The listing builds one solid part. Answer for the finished solid, in the listing's coordinates (mm). Face numbers are marked on the shaded views. A direction names the side the tool comes from. Coordinates: 2 decimals unless noted, no trailing zeros. Order: outer loops, then holes, each group sorted by start corner. A loop starts at its lowest first (then second) coordinate and runs counter-clockwise, first axis right, second up. Notation, with made-up numbers: (42.25, 60) -> (77.25, 60) arc R11 cw to (77.25, 79) -> close; hole circle Ø7 at (55.5, 38.25). An arc over 180 degrees is marked (long way). Return JSON: item names as keys, results as strings.
from build123d import *

# Parameters (mm, degrees)
F0_R     = 19.05
F2_DEPTH = 6.35
F1_R     = 3.175
F3_DEPTH = 19.05
F4_R     = 3.302
F5_DEPTH = 25.4


with BuildPart() as f2:
    # F0 (on Front) → F2 (new body)
    with BuildSketch(Plane.XZ):
        Circle(F0_R)
    extrude(amount=F2_DEPTH)

    # F1 (on Front) → F3 (join)
    with BuildSketch(Plane.XZ):
        with Locations((4.173186, 11.943939)):
            Circle(F1_R)
        with Locations((-11.943939, 4.173186)):
            Circle(F1_R)
        with Locations((-4.173186, -11.943939)):
            Circle(F1_R)
        with Locations((11.943939, -4.173186)):
            Circle(F1_R)
    extrude(amount=F3_DEPTH)

    # F4 (on face) → F5 (cut)
    with BuildSketch(Plane.XZ.offset(6.35)):
        Circle(F4_R)
    extrude(amount=-F5_DEPTH, mode=Mode.SUBTRACT)


solid = f2.part
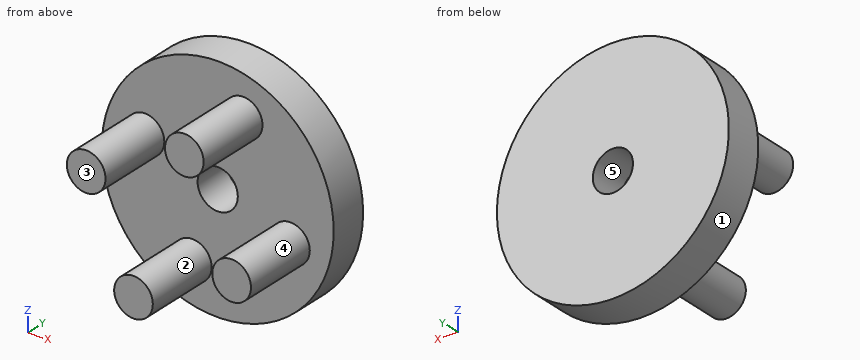
1. The part is cut by section D-D on x = 6.5. Give the vertices of the cut face in (y, z).
Answer block:
{"outline": "(-19.05, 9.78) -> (-6.35, 9.78) -> (-6.35, -17.91) -> (0, -17.91) -> (0, 17.91) -> (-6.35, 17.91) -> (-6.35, 14.1) -> (-19.05, 14.1) -> close"}
2. The part is cut by section B-B on z = 0. Give the vertices of the cut face in (x, y), and give its area (3 significant figures).
Answer block:
{"outline": "(-19.05, -6.35) -> (-3.3, -6.35) -> (-3.3, 0) -> (-19.05, 0) -> close; (3.3, -6.35) -> (19.05, -6.35) -> (19.05, 0) -> (3.3, 0) -> close", "area": "200 mm2"}
3. For the marked faces 1 and 2, determine the directions among +Z, -Z, +X, -X, +Y, -Y from which every point of the face is accessible in a straight line to the end or side of a thin tool.
Answer block:
{"face 1": "+Y, -Y", "face 2": "-Y"}
4. Consider line 1 (Z direction, x = 0, y = -2); line 2 (Y direction, x = 2.5, z = -13); line 3 (X direction, y = -10.75, z = 4). Determine where each line is inside the solid, lowest interval first. Write a range as from..to.
Answer block:
{"line 1": "z = -19.05..-3.3, 3.3..19.05", "line 2": "y = -6.35..0", "line 3": "x = -15.11..-8.77"}
5. The part is cut by section C-C on y = -3.5. Give the vertices of the cut face in (x, z), and give its area (3 significant figures).
Answer block:
{"outline": "circle Ø38.1 at (0, 0); hole circle Ø6.6 at (0, 0)", "area": "1,110 mm2"}
6. The part is cut by section A-A on x = 0. Give the vertices of the cut face in (y, z), and give its area (3 significant figures).
Answer block:
{"outline": "(-6.35, -19.05) -> (0, -19.05) -> (0, -3.3) -> (-6.35, -3.3) -> close; (-6.35, 3.3) -> (0, 3.3) -> (0, 19.05) -> (-6.35, 19.05) -> close", "area": "200 mm2"}
7. Determine the mould class of the marked faces 3, 4 and 5 for opening direction X: pulls with the +X half, pulls with the -X half, needs draft (parallel to the pull), parting line crosses it, or undercut.
Answer block:
{"face 3": "needs draft", "face 4": "parting line crosses it", "face 5": "undercut"}
8. Each of these flat-tipped pins is pushed along its axis until it touches: pin 1 Ø3 at (y, z) = (-16.5, -12.5) entering from -X; pin 2 Ø1.5 at (x, z) = (-1, 4) entering from -Y; pin 3 Ø1 at (y, z) = (-2, 1.5) entering from -X; pin 4 Ø1 at (x, z) = (-12.5, 4) entering from +Y. Where does it stop, or does it pass through?
Answer block:
{"pin 1": "stops at x = -7.35", "pin 2": "stops at y = -6.35", "pin 3": "stops at x = -19.02", "pin 4": "stops at y = 0"}
